Build history of the part. All positions in model axes, mm. Give positions to 0.01 mm unless a question says otherwise; leave off trailing zeros. Return JSON: item names as keys, results as strings. Group by question number.
Q1. Wall check: probe 1 along Z at (x, y) = (180, 2.25); probe 2 along X at (y, z) = (6.75, -30); probe 3 along X at (y, z) = (2.25, -31). Give the ranges that are in metal, low to high.
Q2. Band-saw the part on D-D, the plane z = -30. Count the separate pieces of the cut face and the enclosed holes in it, then the cut area to 3 significant figures.
Q3. Flat gauge pins, fed straight in: pin 1 Ø1.5 at (y, z) = (7.5, -33) entering from +X; pin 2 Ø2 at (x, z) = (158, -38.5) entering from +Y; pin 3 Ø0.8 at (x, y) = (70, 1) entering from +Z. Where does each tip first touch, or does it go through?
Q4. Pull direction X, two halves, no side cores. Call faces 1 (the cylindrical face through (203.5, 6.07, -30.42)), 2 (the cylindrical face through (-3.5, 6.07, -29.58)), 3 (the cylindrical face through (189.237, 4.93, -33.83)), 4 (the flat face through (92, 2.5, 1)): +X half, -X half, draft (parallel to the pull), parting line (faces both ways), or undercut.
Autodesk Inventor part; units mm, degrees
ref_plane "YZ Plane" through (0, 0, 0) normal (1, 0, 0) x (0, 1, 0)
ref_plane "XZ Plane" through (0, 0, 0) normal (0, 1, 0) x (-1, 0, 0)
ref_plane "XY Plane" through (0, 0, 0) normal (0, 0, 1) x (1, 0, 0)
sketch "Sketch1" plane through (0, 0, 0) normal (0, 1, 0) x (-1, 0, 0)
  line L0 (0, 0) -> (-200, 0)
  line L1 (-200, 0) -> (-200, -60)
  line L2 (-200, -60) -> (0, -60)
  line L3 (0, -60) -> (0, 0)
  dimension "d0" = 200
  dimension "d1" = 60
extrude "Extrusion1" add sketch "Sketch1" along normal blind 2.5
sketch "Sketch2" plane through (0, 0, 0) normal (0, -1, 0) x (1, 0, 0)
  line L0 (200, 0) -> (200, -60)
  line L1 (200, 0) -> (180, 0)
  line L2 (180, 0) -> (180, -30)
  line L3 (180, -30) -> (200, -30)
  line L4 (200, -30) -> (200, 0)
  circle A0 centre (180, -30) radius 10
  line L5 (0, 0) -> (200, 0)
  line L6 (180, -30) -> (140, -30)
  line L7 (140, -30) -> (140, 0)
  line L8 (140, 0) -> (180, 0)
  line L9 (180, 0) -> (180, -30)
  circle A1 centre (140, -30) radius 10
  dimension "d4" = 20
  dimension "d5" = 30
  dimension "d6" = 20
  dimension "d7" = 40
sketch "Sketch4" plane through (0, 2.5, 0) normal (0, 1, 0) x (1, 0, 0)
  line L0 (0, 0) -> (200, 0)
  line L1 (200, 0) -> (200, -5)
  line L2 (200, -5) -> (0, -5)
  line L3 (0, -5) -> (0, 0)
  line L4 (0, -5) -> (-5, -5)
  line L5 (-5, -5) -> (-5, 65)
  line L6 (-5, 65) -> (0, 65)
  line L7 (0, 65) -> (0, -5)
  line L8 (0, 60) -> (0, 0)
  line L9 (0, 0) -> (200, 0)
  line L10 (200, 0) -> (200, 65)
  line L11 (200, 65) -> (0, 65)
  line L12 (0, 65) -> (0, 0)
  line L13 (200, 65) -> (205, 65)
  line L14 (205, 65) -> (205, -5)
  line L15 (205, -5) -> (200, -5)
  line L16 (200, -5) -> (200, 65)
  dimension "d8" = 200
  dimension "d9" = 5
  dimension "d10" = 5
  dimension "d11" = 70
  dimension "d12" = 5
extrude "Extrusion2" add sketch "Sketch4" along normal blind 5
extrude "Extrusion3" cut sketch "Sketch2" against normal blind 7.5 contours A0 L6 L3 | L3 L2 A0 | L2 L6 A0 | A1 L6 L7 | L7 L6 A1
fillet "Fillet1" radius 5 4 edges at (205, 5, 5) (205, 5, -65) (-5, 5, -65) (-5, 5, 5)
fillet "Fillet2" radius 5 7 edges at (-3.5355, 7.5, 3.5355) (100, 7.5, 5) (203.5355, 7.5, 3.5355) (205, 7.5, -30) (203.5355, 7.5, -63.5355) (-3.5355, 7.5, -63.5355) (-5, 7.5, -30)
sketch "Sketch5" plane through (0, 0, 0) normal (0, -1, 0) x (1, 0, 0)
  line L0 (0, 0) -> (200, 0)
  line L1 (200, -60) -> (0, -60)
  line L2 (0, 0) -> (50, 0)
  line L3 (50, 0) -> (50, -60)
  line L4 (50, -60) -> (0, -60)
  line L5 (0, -60) -> (0, 0)
  circle A0 centre (50, -30) radius 12.5
  dimension "d19" = 50
  dimension "d20" = 25
extrude "Extrusion4" cut sketch "Sketch5" against normal blind 7.5 contours A0 L3 | L3 A0
sketch "Sketch6" plane through (0, 7.5, 0) normal (0, 1, 0) x (1, 0, 0)
  circle A0 centre (50, 30) radius 12.5
  circle A1 centre (50, 30) radius 15
  circle A2 centre (140, 30) radius 10
  circle A3 centre (140, 30) radius 12.5
  circle A4 centre (180, 30) radius 10
  circle A5 centre (180, 30) radius 12.5
  point P0 (0, 0)
  dimension "d23" = 30
  dimension "d24" = 25
extrude "Extrusion5" add sketch "Sketch6" along normal blind 2.5
fillet "Fillet3" radius 2.5 3 edges at (127.5, 10, -30) (167.5, 10, -30) (35, 10, -30)
properties part number "Cover"
From the geometry:
{
 "1": {"probe 1": "z = -60 to -40, -20 to 0", "probe 2": "x = -2.63 to 37.5, 62.5 to 130, 150 to 170, 190 to 202.63", "probe 3": "x = 0 to 37.54, 62.46 to 130.05, 149.95 to 170.05, 189.95 to 200"},
 "2": {"separate pieces": "4", "enclosed holes": "0", "area": "1,080 mm^2"},
 "3": {"pin 1": "stops at x = 202.63", "pin 2": "stops at y = 7.5", "pin 3": "stops at z = 0"},
 "4": {"face 1": "+X half", "face 2": "-X half", "face 3": "undercut", "face 4": "draft"}
}
